Could you check a few things on this model? Use its own coordinates, in mm. Face numbers are marked on the shaded views. A direction names the side the tool comes from. Give positions to 0.01 mm unless a question says otherwise; leave off trailing zeros. Use a Markdown table: item, result. Add a question column.
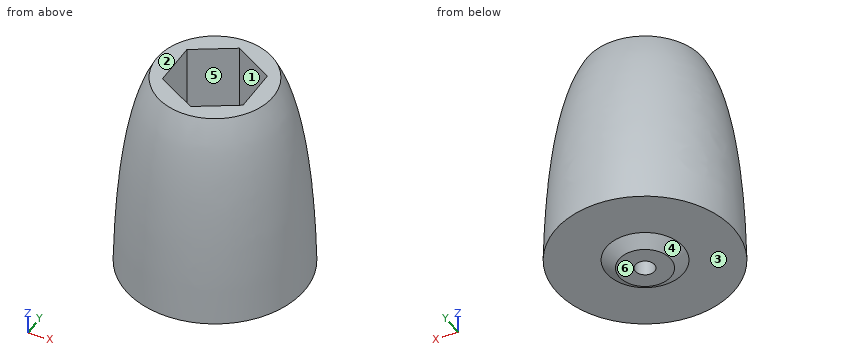
```python
from build123d import *

# Parameters (mm, degrees)
F3_DEPTH = 6
F4_R     = 0.75
F5_DEPTH = 10.691096


with BuildPart() as f1:
    # F0 (on Front) → F1 (revolve)
    with BuildSketch(Plane.XZ):
        with BuildLine():
            Line((0, -0.690096), (0, 0))
            Line((0, 0), (0, 16))
            Line((0, 16), (-4.5, 16))
            add(Edge.make_bspline(
                [(-4.5, 16), (-6.14538, 12.944644), (-6.807135, 6.615023), (-6.95, 0)],
                knots=[0, 0, 0, 0, 16.186491, 16.186491, 16.186491, 16.186491], degree=3))
            Line((-6.95, 0), (-3, 0))
            Line((-3, 0), (-2.014441, -0.690096))
            Line((-2.014441, -0.690096), (0, -0.690096))
        make_face()
    revolve(axis=Axis((0, 0, 8), (0, 0, 1)))

    # F2 (on face) → F3 (cut)
    with BuildSketch(Plane.XY.offset(16)):
        Polygon((-0.037923, 3.579371), (-3.118788, 1.756843), (-3.080864, -1.822528), (0.037923, -3.579371), (3.118788, -1.756843), (3.080864, 1.822528), align=None)
    extrude(amount=-F3_DEPTH, mode=Mode.SUBTRACT)

    # F4 (on face) → F5 (cut, through all)
    with BuildSketch(Plane.XY.offset(10)):
        Circle(F4_R)
    extrude(amount=-F5_DEPTH, mode=Mode.SUBTRACT)


solid = f1.part
```
1) For the marked faces 1, 2 and 3, which set-ups out of +Z, -Z, +X, -X, +Y, -Y let a thin tool reach every point of the face, with its end or its side?
2) We'd pull the mould along X, two halves only. Please class the marked faces 4, 5 and 6: pulls with the +X half, pulls with the -X half, needs draft (parallel to the pull), parting line crosses it, or undercut.
3) For pin 1 (3 mm diameter, centred on x = 2, z = 5, fed in from +Y); pin 2 (2 mm diameter, centred on x = -3, z = 9.5, fed in from -Y); pin 3 (3 mm diameter, centred on x = 5.5, z = 13, fed in from +Y), each with a flat end and sliding along its axis, tell me the tip position at first contact or that it passes through.
4) Please list where these lines run through material, in increasing order: line 1 (Y direction, x = 0, z = 3.5); line 2 (Y direction, x = 0, z = 5); line 3 (Z direction, x = -1.5, y = -0.5). Write a range as from..to.
Values found:
| question | item | result |
|---|---|---|
| 1 | face 1 | +Z |
| 1 | face 2 | +Z, +X, -X, +Y, -Y |
| 1 | face 3 | -Z |
| 2 | face 4 | parting line crosses it |
| 2 | face 5 | undercut |
| 2 | face 6 | needs draft |
| 3 | pin 1 | stops at y = 6.74 |
| 3 | pin 2 | stops at y = -5.97 |
| 3 | pin 3 | stops at y = 4 |
| 4 | line 1 | y = -6.82..-0.75, 0.75..6.82 |
| 4 | line 2 | y = -6.73..-0.75, 0.75..6.73 |
| 4 | line 3 | z = -0.69..10 |
